The listing builds one solid part. Answer for the finished solid, in the listing's coordinates (mm). A direction names the side the tool comes from. Coordinates: 2 decimals unless noted, no trailing zeros. Write each loop counter-clockwise with the first axis right and the second up, starting at its lowest first coordinate (ties: lowest second). Pieces come first, ordered by that corner, then holes.
from build123d import *

# Parameters (mm, degrees)
ESBO_O2_R                = 0.75
RESSALTO_EXTRUS_O1_DEPTH = 2
PADR_OCIRCULAR1_COUNT    = 6
ESBO_O3_R                = 4
ESBO_O3_R_2              = 2.5
RESSALTO_EXTRUS_O2_DEPTH = 3.5
CORTE_EXTRUS_O1_START    = -1
ESBO_O4_R                = 2.5
ESBO_O4_R_2              = 0.75
CORTE_EXTRUS_O1_DEPTH    = 1
RESSALTO_EXTRUS_O3_START = 1
ESBO_O5_R                = 3
ESBO_O5_R_2              = 2.5
RESSALTO_EXTRUS_O3_DEPTH = 1


with BuildPart() as part:
    # Esboço2 → Ressalto-extrusão1 (new body)
    with BuildSketch(Plane(origin=(0, 0, 0), x_dir=(1, 0, 0), z_dir=(0, 1, 0))):
        with BuildLine():
            Line((-13.672903959, 1.992512038), (-4.128356106, 2.82075803))
            ThreePointArc((-4.128356106, 2.82075803), (5, 0), (-4.128356106, -2.82075803))
            Line((-4.128356106, -2.82075803), (-13.672903959, -1.992512038))
            ThreePointArc((-13.672903959, -1.992512038), (-15.5, 0), (-13.672903959, 1.992512038))
        make_face()
        with Locations(Location((0, 0, 0), (0, 0, 270))):
            Circle(ESBO_O2_R, mode=Mode.SUBTRACT)
        with Locations(Location((-7, 0, 0), (0, 0, 270))):
            Circle(ESBO_O2_R, mode=Mode.SUBTRACT)
        with Locations(Location((-10.25, 0, 0), (0, 0, 270))):
            Circle(ESBO_O2_R, mode=Mode.SUBTRACT)
        with Locations(Location((-13.5, 0, 0), (0, 0, 270))):
            Circle(ESBO_O2_R, mode=Mode.SUBTRACT)
    ressalto_extrus_o1 = extrude(amount=RESSALTO_EXTRUS_O1_DEPTH)

    # PadrãoCircular1: Ressalto-extrusão1 ×6 about axis
    padr_ocircular1_axis = Axis((0, 0, 0), (0, 1, 0))
    for i in range(1, PADR_OCIRCULAR1_COUNT):
        add(ressalto_extrus_o1.rotate(padr_ocircular1_axis, i * 360 / PADR_OCIRCULAR1_COUNT))

    # Esboço3 → Ressalto-extrusão2 (add)
    with BuildSketch(Plane(origin=(0, 2, 0), x_dir=(1, 0, 0), z_dir=(0, 1, 0))):
        with Locations(Location((0, 0, 0), (0, 0, 270))):
            Circle(ESBO_O3_R)
        with Locations(Location((0, 0, 0), (0, 0, 270))):
            Circle(ESBO_O3_R_2, mode=Mode.SUBTRACT)
    extrude(amount=RESSALTO_EXTRUS_O2_DEPTH)

    # Esboço4 → Corte-extrusão1 (cut)
    with BuildSketch(Plane(origin=(0, 2, 0), x_dir=(1, 0, 0), z_dir=(0, 1, 0)).offset(CORTE_EXTRUS_O1_START)):
        with Locations(Location((0, 0, 0), (0, 0, 270))):
            Circle(ESBO_O4_R)
        with Locations(Location((0, 0, 0), (0, 0, 270))):
            Circle(ESBO_O4_R_2, mode=Mode.SUBTRACT)
    extrude(amount=CORTE_EXTRUS_O1_DEPTH, mode=Mode.SUBTRACT)

    # Esboço5 → Ressalto-extrusão3 (add)
    with BuildSketch(Plane.XZ.offset(RESSALTO_EXTRUS_O3_START)):
        with Locations(Location((0, 0, 0), (0, 0, 90))):
            Circle(ESBO_O5_R)
        with Locations(Location((0, 0, 0), (0, 0, 90))):
            Circle(ESBO_O5_R_2, mode=Mode.SUBTRACT)
    extrude(amount=-RESSALTO_EXTRUS_O3_DEPTH)


solid = part.part
1. Flat-ended cylindrical pins translate along their axes: P1, Ø2.5, axis at x = -6.75, z = -11.69, coming from the +Y side; P2, Ø1.5, axis at y = 2, z = -8, coming from the -X side; P3, Ø2, axis at x = 0, z = 0, coming from the -Y side. Find the tip coordinate at first contact, or state that the pin passes through.
Results found:
P1: stops at y = 2
P2: stops at x = -7.58
P3: stops at y = 0
2. A tool of negligible diameter and unlimited length cuts with its end or side. For faces 1 (the flat face through (2, 5.5, 2)), 2 (the cylindrical face through (-0.9, -0.51, 2.86)), 3 (the flat face through (6.65, 0.99, 6.75)), 4 (the flat face through (-9.292, 0.986, -2.373)), 5 (the cylindrical face through (-4.244, 0.986, 6.16)), from which of +Z, -Z, +X, -X, +Y, -Y can it reach the whole face along a straight path? Write none if from no direction.
Results found:
face 1: +Z, -Z, +X, -X, +Y
face 2: -Y
face 3: +X, +Y, -Y
face 4: -X, +Y, -Y
face 5: +Y, -Y
3. Section C-C on x = 10.25 is taken. Give the vertices of the cut face in (y, z).
Results found:
outline: (0, -2.29) - (2, -2.29) - (2, -0.75) - (0, -0.75) - close; (0, 0.75) - (2, 0.75) - (2, 2.29) - (0, 2.29) - close
4. Section D-D on y = 3.75 is taken. Give the vertices of the cut face in (x, z), then the cut area to 3 significant figures.
Results found:
outline: circle Ø8 at (0, 0); hole circle Ø5 at (0, 0)
area: 30.6 mm2
5. Section B-B on x = 3.5 is taken. Give the vertices of the cut face in (y, z).
Results found:
outline: (0, -10.53) - (2, -10.53) - (2, -6.81) - (0, -6.81) - close; (0, -5.31) - (2, -5.31) - (2, -1.94) - (5.5, -1.94) - (5.5, 1.94) - (2, 1.94) - (2, 5.31) - (0, 5.31) - close; (0, 6.81) - (2, 6.81) - (2, 10.53) - (0, 10.53) - close
6. For a pull along Z with two mould halves and no side action, classify faces 6 (the cylindrical face through (7.29, 0.99, -0.69)), 7 (the flat face through (-2.5, 1, 9.1)), 8 (the cylindrical face through (-3.533, 0.986, -5.313)), 9 (the cylindrical face through (-3.905, 3.726, -0.867)) as pulls with the +Z half, pulls with the -Z half, needs draft (parallel to the pull), parting line crosses it, or undercut.
Results found:
face 6: undercut
face 7: pulls with the +Z half
face 8: undercut
face 9: parting line crosses it
7. Find the intervals of material crossed by L1, parallel to X at y = -0.3, z = 0; L2, parallel to X at y = 1, z = 8.25; L3, parallel to Y at x = -3.5, z = -10, in increasing order.
Results found:
L1: x = -3 to -2.5, 2.5 to 3
L2: x = -7.35 to -5.54, -4.71 to -1.9, 1.9 to 4.71, 5.54 to 7.35
L3: y = 0 to 2
8. Section A-A on z = 7.5 is taken. Give the vertices of the cut face in (x, y), then the cut area to 3 significant figures.
Results found:
outline: (-7, 0) - (-1.38, 0) - (-1.38, 2) - (-7, 2) - close; (1.38, 0) - (7, 0) - (7, 2) - (1.38, 2) - close
area: 22.5 mm2
